Can you work these out from the drawing? Everything is in mm from the part's minimum corner. A direction names the side the tool comes from. Give positions to 0.01 mm unless a question says otherwise; leave off trailing zeros. Order: outer loops, then holes, each group sorted by start corner. A loop starts at its lowest first (then second) coordinate and runs counter-clockwise, first axis right, second up. Notation, with made-up numbers: M -37.75,37 L 4.25,37 A28 ccw 4.25,71 Z; hole C -36,23.5 d2. An arc over 180 degrees is marked long. Use a Markdown table: item, result. Add a question column.
Item 1: If I drill on L1, parallel to Z at x = 10.5, y = 56; L2, parallel to Z at x = 58.5, y = 12.5 (1 decimal); L3, parallel to X at y = 23, z = 35.5, over which ranges is the centre line in solid material (lowest first)? Write a range as from..to.
Item 2: I'm going to push flat-ended pins straight in: pin 1 Ø3 at (x, z) = (67.5, 22) entering from -Y; pin 2 Ø10 at (x, y) = (53.5, 19.5) entering from +Z (1 decimal); pin 3 Ø10 at (y, z) = (17.5, 31.5) entering from +X (1 decimal); pin 4 Ø10 at (x, y) = (58.5, 28) entering from +Z. Where does each tip first touch, or does it pass through?
Item 3: Suppose I cut it at A-A on y = 14. Write out the boundary of the cut face in (x, z) (1 decimal), plus the area to 3 significant figures.
Item 4: Suppose I cut it at B-B on x = 52. Write out the boundary of the cut face in (y, z) (1 decimal).
Item 5: Suppose I cut it at C-C on z = 30. Write out the boundary of the cut face in (x, y) (1 decimal), plus the area to 3 significant figures.
Item 6: Suppose I cut it at D-D on x = 80. Write out the boundary of the cut face in (y, z), plus the area to 3 significant figures.
Item 7: For the marked faces 1 and 2, which set-ups out of +Z, -Z, +X, -X, +Y, -Y let a thin tool reach every point of the face, with its end or its side?
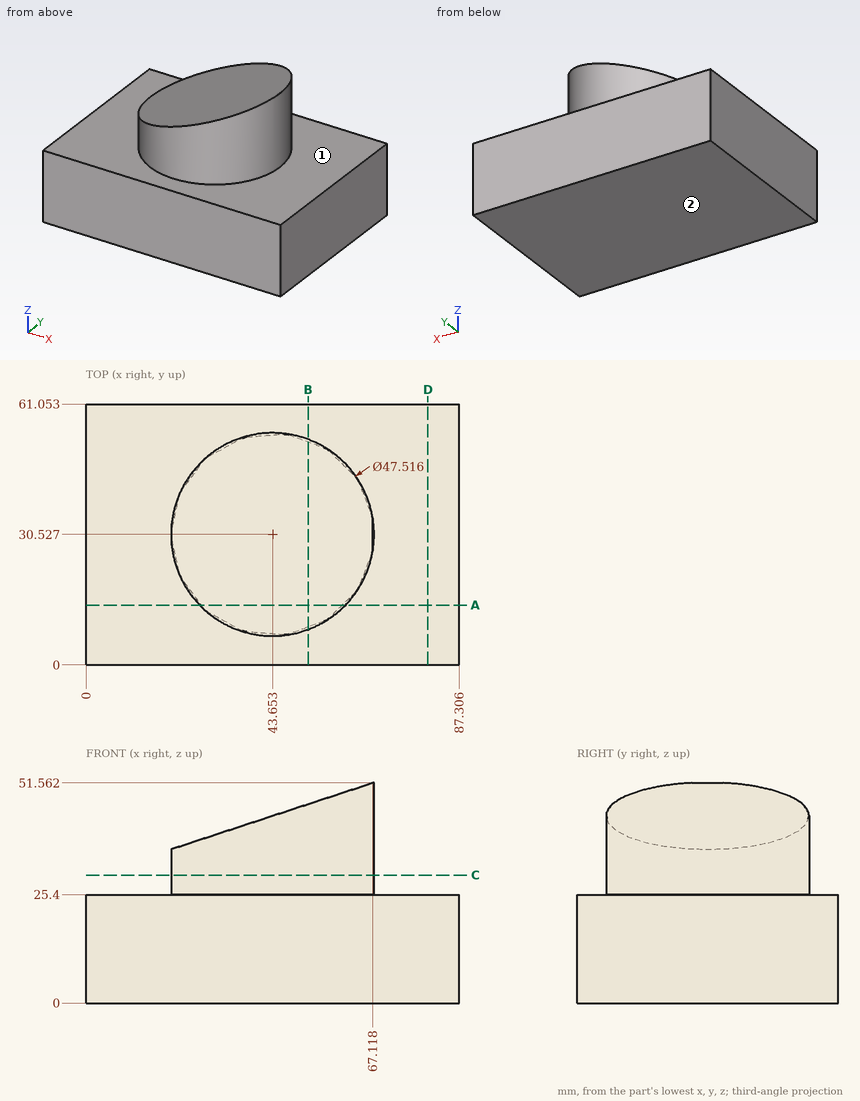
Findings below:
| question | item | result |
|---|---|---|
| 1 | L1 | z = 0..25.4 |
| 1 | L2 | z = 0..48.7 |
| 1 | L3 | x = 21.12..66.19 |
| 2 | pin 1 | stops at y = 0 |
| 2 | pin 2 | stops at z = 48.7 |
| 2 | pin 3 | stops at x = 66 |
| 2 | pin 4 | stops at z = 50.37 |
| 3 | outline | M 0,0 L 87.3,0 L 87.3,25.4 L 60.7,25.4 L 60.7,49.5 L 26.6,38.2 L 26.6,25.4 L 0,25.4 Z |
| 3 | area | 2,850 mm^2 |
| 4 | outline | M 0,0 L 61.1,0 L 61.1,25.4 L 52.8,25.4 L 52.8,46.6 L 8.3,46.6 L 8.3,25.4 L 0,25.4 Z |
| 5 | outline | C 43.7,30.5 d47.5 |
| 5 | area | 1,770 mm^2 |
| 6 | outline | M 0,0 L 61.05,0 L 61.05,25.4 L 0,25.4 Z |
| 6 | area | 1,550 mm^2 |
| 7 | face 1 | +Z |
| 7 | face 2 | -Z, +X, -X, +Y, -Y |
